Here's how the part is built. I have some questions about the finished solid (model axes, mm). Face numbers are marked on the shaded views. A direction names the side the tool comes from. Give positions to 0.01 mm unless a question says otherwise; leave off trailing zeros. Loops run counter-clockwise (first coordinate to the right, second up) from the corner with the lowest first, then second, coordinate; pieces in that order, holes last. Notation, with made-up numbers: (17.25, 0.25) - (76.25, 0.25) arc R13 ccw to (76.25, 14.25) - close; hole circle Ø7 at (2, 0). An arc over 180 degrees is marked (long way). Return JSON: item names as keys, results as strings. Group by question number.
(1) If we mould it in two halves opening along Y, with no side actions, what happens to the marked faces 1, 2 and 3? For each: released by +Y, released by -Y, zero draft, split by the parting line, or undercut.
(2) On a 3-axis mill with a long thin cutter (end or side, diameter ignored), from which of +Z, -Z, +X, -X, +Y, -Y can I reach the whole of each face in a straight line? I mean the marked faces 4, 5 and 6. Say none if no direction works.
(3) I need wall thicknesses on probe 1 along Z at (x, y) = (0, -3.65); probe 2 along Y at (x, z) = (17.5, 11.5); probe 3 along Y at (x, z) = (21.5, 2). Which ranges of each line are inside material? Lowest first, please. Write a range as [from, to].
(4) If we section it at C-C (z = 7.5): State how many separate pieces and enclosed holes the cut face has, then the cut area to 3 significant figures.
(5) For P1, Ø4.5, axis at y = 8, z = 8.5, coming from the +X side; P2, Ø1.5, axis at x = -18, y = -9, coming from the -Z side; P3, Ø2, axis at y = 13, z = 6, coming from the -X side, each with a flat end and sliding along its axis, tell me the tip position at first contact or that it passes through.
(6) If we section it at D-D (y = -6): Please give me the cut outline in (x, z).
(7) If we section it at A-A (y = 1.5): Please give me the cut outline in (x, z), then the cut area to 3 significant figures.
```python
from build123d import *

# Parameters (mm, degrees)
F1_DEPTH = 23.3
F2_W     = 30
F2_H     = 8.6
F3_DEPTH = 5
F4_R     = 3
F5_DEPTH = 2
F7_DEPTH = 10
F8_W     = 12
F8_H     = 1
F9_DEPTH = 35.801
F10_R    = 0.49999


# Not quite as in the source:
# - a fillet or chamfer is up to 0.001 mm smaller than in the source, because OpenCascade refuses the exact size


with BuildPart() as f1:
    # F0 (on Right) → F1 (new body, symmetric)
    with BuildSketch(Plane.YZ):
        Polygon((-5, 12), (-5, 0), (0, 0), (0, 15), (-10, 15), (-10, 6.4), (-7, 6.4), (-7, 12), align=None)
    extrude(amount=F1_DEPTH, both=True)

    # F2 (on face) → F3 (cut, through all)
    with BuildSketch(Plane.XZ.offset(10)):
        with Locations((0, 10.7)):
            Rectangle(F2_W, F2_H)
    extrude(amount=-F3_DEPTH, mode=Mode.SUBTRACT)

    # F4 (on face) → F5 (cut)
    with BuildSketch(Plane.XZ.offset(5)):
        with Locations((0, 7.5)):
            Circle(F4_R)
    extrude(amount=-F5_DEPTH, mode=Mode.SUBTRACT)

    # F6 (on face) → F7 (join)
    with BuildSketch(Plane.XY.offset(15)):
        Polygon((-12.5, 16), (-12.5, 0), (-9.5, 0), (-9.5, 13), (-9.5, 16), align=None)
        Polygon((9.5, 13), (9.5, 0), (12.5, 0), (12.5, 16), (9.5, 16), align=None)
    extrude(amount=-F7_DEPTH)

    # F8 (on face) → F9 (cut, through all)
    with BuildSketch(Plane.YZ.offset(12.5)):
        with Locations((6, 14.5)):
            Rectangle(F8_W, F8_H)
    extrude(amount=-F9_DEPTH, mode=Mode.SUBTRACT)

    # F10 (radius 0.5 in the source; OpenCascade refuses exactly that, so slightly less here)
    f10_edges = [f1.edges().sort_by_distance(p)[0] for p in [
        (-9.5, 6, 14),
        (-9.5, 12, 14.5),
        (-9.5, 14, 15),
        (-9.5, 16, 10),
        (-9.5, 8, 5),
        (-9.5, 0, 9.5),
        (12.5, 6, 14),
        (12.5, 12, 14.5),
        (12.5, 14, 15),
        (12.5, 16, 10),
        (12.5, 8, 5),
        (12.5, 0, 9.5),
        (9.5, 14, 15),
        (9.5, 12, 14.5),
        (9.5, 6, 14),
        (9.5, 0, 9.5),
        (9.5, 8, 5),
        (9.5, 16, 10),
        (-12.5, 14, 15),
        (-12.5, 12, 14.5),
        (-12.5, 6, 14),
        (-12.5, 0, 9.5),
        (-12.5, 8, 5),
        (-12.5, 16, 10),
        (11, 12, 14),
        (-11, 12, 14),
        (-11, 16, 15),
        (-11, 12, 15),
        (11, 16, 15),
        (11, 12, 15),
        (0, 0, 0),
        (-23.3, 0, 7.5),
        (0, 0, 15),
        (23.3, 0, 7.5),
        (11, 0, 14),
        (11, 0, 5),
        (-11, 0, 14),
        (-11, 0, 5),
    ]]
    fillet(f10_edges, radius=F10_R)


solid = f1.part
```
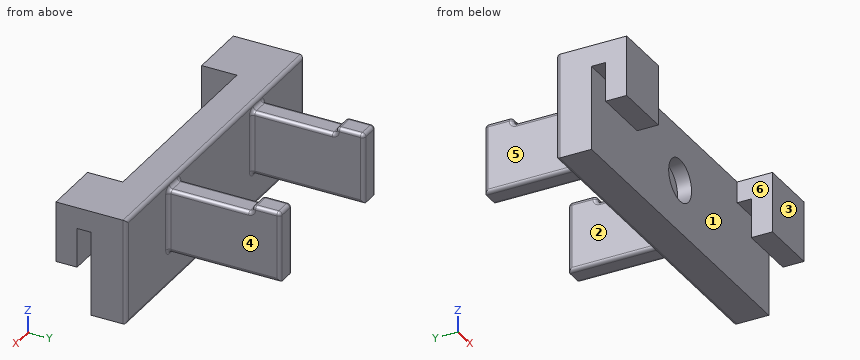
Values:
{
 "1": {"face 1": "undercut", "face 2": "zero draft", "face 3": "released by -Y"},
 "2": {"face 4": "+Z, -Z, +X, +Y", "face 5": "+Z, -Z, -X, +Y", "face 6": "+Z, -Z, -Y"},
 "3": {"probe 1": "[0, 4.5], [10.5, 15]", "probe 2": "[-10, -7], [-5, 0]", "probe 3": "[-5, 0]"},
 "4": {"separate pieces": "3", "enclosed holes": "0", "area": "367 mm2"},
 "5": {"P1": "x = 12.5", "P2": "z = 6.4", "P3": "x = -12.5"},
 "6": {"outline": "(-23.3, 12) - (-15, 12) - (-15, 15) - (-23.3, 15) - close; (15, 12) - (23.3, 12) - (23.3, 15) - (15, 15) - close"},
 "7": {"outline": "(-12.5, 5.5) arc R0.5 ccw to (-12, 5) - (-10, 5) arc R0.5 ccw to (-9.5, 5.5) - (-9.5, 13.5) arc R0.5 ccw to (-10, 14) - (-12, 14) arc R0.5 ccw to (-12.5, 13.5) - close; (9.5, 5.5) arc R0.5 ccw to (10, 5) - (12, 5) arc R0.5 ccw to (12.5, 5.5) - (12.5, 13.5) arc R0.5 ccw to (12, 14) - (10, 14) arc R0.5 ccw to (9.5, 13.5) - close", "area": "53.6 mm2"}
}
